```python
from build123d import *

# Parameters (mm, degrees)
ESQUISSE1_W             = 40
ESQUISSE1_H             = 20
BOSS_EXTRU_1_DEPTH      = 42.5
BOSS_EXTRU_2_DEPTH      = 7
BOSS_EXTRU_2_DEPTH_BACK = 48
ESQUISSE2_W             = 2
ESQUISSE2_H             = 20
ESQUISSE3_R             = 2
ENL_V_MAT_EXTRU_1_DEPTH = 7.5
ESQUISSE5_R             = 2.65
BOSS_EXTRU_3_DEPTH      = 3


with BuildPart() as part:
    # Esquisse1 → Boss.-Extru.1 (new body)
    with BuildSketch(Plane.XY):
        with Locations((10, 0)):
            Rectangle(ESQUISSE1_W, ESQUISSE1_H)
    extrude(amount=-BOSS_EXTRU_1_DEPTH)

    # Esquisse2 → Boss.-Extru.2 (add, two sides: drawn at the far end of the back side and taken through both)
    with BuildSketch(Plane(origin=(30, 0, 0), x_dir=(0, 0, -1), z_dir=(1, 0, 0)).offset(-BOSS_EXTRU_2_DEPTH_BACK)):
        with Locations((10.5, 0)):
            Rectangle(ESQUISSE2_W, ESQUISSE2_H)
    extrude(amount=BOSS_EXTRU_2_DEPTH + BOSS_EXTRU_2_DEPTH_BACK)

    # Esquisse3 → Enlèv. mat.-Extru.1 (cut)
    with BuildSketch(Plane(origin=(0, 0, -11.5), x_dir=(-1, 0, 0), z_dir=(0, 0, -1))):
        with Locations(Location((14, 5, 0), (0, 0, 270))):
            Circle(ESQUISSE3_R)
        with Locations((14, -5)):
            Circle(ESQUISSE3_R)
        with Locations(Location((-34, -5, 0), (0, 0, 270))):
            Circle(ESQUISSE3_R)
        with Locations((-34, 5)):
            Circle(ESQUISSE3_R)
    extrude(amount=-ENL_V_MAT_EXTRU_1_DEPTH, mode=Mode.SUBTRACT)

    # Esquisse5 → Boss.-Extru.3 (add)
    with BuildSketch(Plane(origin=(0, 0, 0), x_dir=(-1, 0, 0), z_dir=(0, 0, -1))):
        Circle(ESQUISSE5_R)
    extrude(amount=-BOSS_EXTRU_3_DEPTH)


solid = part.part
```
Work out the finished part from the listing and answer in its coordinate system (mm). A direction names the side the tool comes from. Coordinates: 2 decimals unless noted, no trailing zeros. Write each loop counter-clockwise with the first axis right and the second up, starting at its lowest first coordinate (ties: lowest second). Pieces come first, ordered by that corner, then holes. Notation, with made-up numbers: (75, -34) - (128, -34) arc R14 cw to (128, -10) - close; hole circle Ø4 at (-25, 59). An arc over 180 degrees is marked (long way). Answer as a JSON object with one key per item and string values.
Q1. Find section A-A (y = 5). Write down the section's boundary in (x, z).
Results list:
{"outline": "(-18, -11.5) - (-16, -11.5) - (-16, -9.5) - (-18, -9.5) - close; (-12, -11.5) - (-10, -11.5) - (-10, -42.5) - (30, -42.5) - (30, -11.5) - (32, -11.5) - (32, -9.5) - (30, -9.5) - (30, 0) - (-10, 0) - (-10, -9.5) - (-12, -9.5) - close; (36, -11.5) - (37, -11.5) - (37, -9.5) - (36, -9.5) - close"}
Q2. Consider L1, parallel to Y at x = -14, z = -10.05; L2, parallel to Z at x = 5, y = -2.5; L3, parallel to X at y = 9.25, z = -4.5. Determine where each line is inside the solid, lowest interval first. Write a range as from..to.
Results list:
{"L1": "y = -10..-7, -3..3, 7..10", "L2": "z = -42.5..0", "L3": "x = -10..30"}
Q3. Find section D-D (y = 0). Write down the section's boundary in (x, z), plus the area to 3 significant figures.
Results list:
{"outline": "(-18, -11.5) - (-10, -11.5) - (-10, -42.5) - (30, -42.5) - (30, -11.5) - (37, -11.5) - (37, -9.5) - (30, -9.5) - (30, 0) - (2.65, 0) - (2.65, 3) - (-2.65, 3) - (-2.65, 0) - (-10, 0) - (-10, -9.5) - (-18, -9.5) - close", "area": "1,750 mm^2"}
Q4. Which of the six approach directions +Z, -Z, +X, -X, +Y, -Y give full straight-line access (tool end or side, diameter ignored) to faces 1 (the cylindrical face through (-2.45, -1.01, 1.48)), 2 (the flat face through (-14, 0, -9.5)), 3 (the flat face through (-10, 0, -27)), 4 (the flat face through (33, 0, -9.5))?
Results list:
{"face 1": "+Z", "face 2": "+Z, -X, +Y, -Y", "face 3": "-Z, -X, +Y, -Y", "face 4": "+Z, +X, +Y, -Y"}
Q5. Given pin 1 Ø1 at (x, y) = (-6.5, -4.5) entering from +Z; pin 2 Ø2 at (x, y) = (35, -3.5) entering from -Z; pin 3 Ø10 at (y, z) = (1, -24.5) entering from +X, each flat-ended and moving along its own axis, determine where each tip first touches the part or whether it passes through.
Results list:
{"pin 1": "stops at z = 0", "pin 2": "stops at z = -11.5", "pin 3": "stops at x = 30"}
Q6. Find section B-B (x = -14). Write down the section's boundary in (y, z), plus the area to 3 significant figures.
Results list:
{"outline": "(-10, -11.5) - (-7, -11.5) - (-7, -9.5) - (-10, -9.5) - close; (-3, -11.5) - (3, -11.5) - (3, -9.5) - (-3, -9.5) - close; (7, -11.5) - (10, -11.5) - (10, -9.5) - (7, -9.5) - close", "area": "24.0 mm^2"}
Q7. Find section C-C (x = 0). Write down the section's boundary in (y, z).
Results list:
{"outline": "(-10, -42.5) - (10, -42.5) - (10, 0) - (2.65, 0) - (2.65, 3) - (-2.65, 3) - (-2.65, 0) - (-10, 0) - close"}
Q8. For a pull along X with two mould halves and no side action, classify faces 5 (the flat face through (30, 0, -5)), 6 (the cylindrical face through (36, -5, -11)), 7 (the flat face through (33, 0, -11.5)) as pulls with the +X half, pulls with the -X half, needs draft (parallel to the pull), parting line crosses it, or undercut.
Results list:
{"face 5": "pulls with the +X half", "face 6": "undercut", "face 7": "needs draft"}
